Work out the finished part from the listing and answer in its coordinate system (mm). A direction names the side the tool comes from. Coordinates: 2 decimals unless noted, no trailing zeros. Write each loop counter-clockwise with the first axis right and the second up, starting at its lowest first coordinate (ties: lowest second). Pieces come first, ordered by that corner, then holes. Notation, with made-up numbers: (70.5, 60.5) - (118.5, 60.5) arc R6 cw to (118.5, 70.5) - close; hole circle Ø11 at (26.5, 38.25). An arc over 180 degrees is marked (long way). Use a Markdown table: item, result. Add a question column.
(1) A tool of negligible diameter and unlimited length cuts with its end or side. For faces 4 (the face through (1, 1, 1)), 5 (the face through (-2, 3.9, 2)), 6 (the face through (0.736, 2.683, 2.337)), from which of +Z, -Z, +X, -X, +Y, -Y can it reach the whole face along a straight path? Write none if from no direction.
(2) For a pull along Z with two mould halves and no side action, classify faces 1 (the face through (7, 0, 0)), 2 (the face through (17.2, 0.7, 0)), 3 (the face through (-1, 1.5, -1)) as released by +Z, released by -Z, zero draft, split by the parting line, or undercut.
(3) The part is cut by section B-B, the plane y = 0.4. State how many separate pieces and enclosed holes the cut face has, then the cut area to 3 significant figures.
(4) Given pin 1 Ø4 at (x, z) = (0, 0) entering from -Y; pin 2 Ø1.8 at (x, z) = (10, 0) entering from +Y; pin 3 Ø1.5 at (x, y) = (7, 1.5) entering from +Z, each flat-ended and moving along its own axis, determine where each tip first touches the part or whether it passes through.
(5) The part is cut by section D-D, the plane z = -1.5. Give the vertices of the cut face in (x, y), then the cut area to 3 significant figures.
(6) Find the intervals of material crossed by line 1 (X direction, y = 2.25, z = 1); line 2 (Y direction, x = 8.75, z = 0); line 3 (X direction, y = 0.65, z = 1.25), in increasing order. Write a range as from..to.
(7) The part is cut by section C-C, the plane z = 1. Give the vertices of the cut face in (x, y), then the cut area to 3 significant figures.
(8) The part is cut by section A-A, the plane x = 9.8. Give the vertices of the cut face in (y, z), then the cut area to 3 significant figures.
from build123d import *

# Parameters (mm, degrees)
SKETCH1_R           = 0.5
BOSS_EXTRUDE1_DEPTH = 1.4
SKETCH2_R           = 2.35
CUT_EXTRUDE1_DEPTH  = 1
SKETCH3_R           = 3.5
SKETCH3_R_2         = 2.45
BOSS_EXTRUDE2_DEPTH = 2.5
SKETCH4_R           = 1.2
CUT_EXTRUDE2_DEPTH  = 20.282440198
SKETCH5_R           = 2.45
SKETCH5_R_2         = 1.2
BOSS_EXTRUDE3_DEPTH = 0.1
SKETCH6_W           = 35.735260114
SKETCH6_H           = 17.672039004
CUT_EXTRUDE4_DEPTH  = 20.513392837
CUT_EXTRUDE5_DEPTH  = 18.980545042
SKETCH8_W           = 0.114102852
SKETCH8_H           = 0.1
CUT_EXTRUDE6_DEPTH  = 0.1


with BuildPart() as part:
    # Sketch1 → Boss-Extrude1 (new body)
    with BuildSketch(Plane(origin=(0, 0, 0), x_dir=(1, 0, 0), z_dir=(0, 1, 0))):
        with BuildLine():
            Line((-15.2, 2), (-2, 2.95))
            Line((-2, 2.95), (-2, 6.35))
            ThreePointArc((-2, 6.35), (0, 8.35), (2, 6.35))
            Line((2, 6.35), (2, 3.5))
            Line((2, 3.5), (15.2, 2))
            ThreePointArc((15.2, 2), (17.2, 0), (15.2, -2))
            Line((15.2, -2), (2, -3.5))
            Line((2, -3.5), (2, -6.35))
            ThreePointArc((2, -6.35), (0, -8.35), (-2, -6.35))
            Line((-2, -6.35), (-2, -2.95))
            Line((-2, -2.95), (-15.2, -2))
            ThreePointArc((-15.2, -2), (-17.2, 0), (-15.2, 2))
        make_face()
        with Locations(Location((0, 6.35, 0), (0, 0, 270))):
            Circle(SKETCH1_R, mode=Mode.SUBTRACT)
        with Locations(Location((0, 4.55, 0), (0, 0, 270))):
            Circle(SKETCH1_R, mode=Mode.SUBTRACT)
        with Locations(Location((0, -4.55, 0), (0, 0, 90))):
            Circle(SKETCH1_R, mode=Mode.SUBTRACT)
        with Locations(Location((0, -6.35, 0), (0, 0, 90))):
            Circle(SKETCH1_R, mode=Mode.SUBTRACT)
        with Locations(Location((-15.2, 0, 0), (0, 0, 270))):
            Circle(SKETCH1_R, mode=Mode.SUBTRACT)
        with Locations(Location((15.2, 0, 0), (0, 0, 270))):
            Circle(SKETCH1_R, mode=Mode.SUBTRACT)
        with Locations(Location((-13.4, 0, 0), (0, 0, 270))):
            Circle(SKETCH1_R, mode=Mode.SUBTRACT)
        with Locations(Location((-11.6, 0, 0), (0, 0, 270))):
            Circle(SKETCH1_R, mode=Mode.SUBTRACT)
        with Locations(Location((-9.8, 0, 0), (0, 0, 270))):
            Circle(SKETCH1_R, mode=Mode.SUBTRACT)
        with Locations(Location((-8, 0, 0), (0, 0, 270))):
            Circle(SKETCH1_R, mode=Mode.SUBTRACT)
        with Locations(Location((-6.2, 0, 0), (0, 0, 270))):
            Circle(SKETCH1_R, mode=Mode.SUBTRACT)
        with Locations(Location((-4.4, 0, 0), (0, 0, 270))):
            Circle(SKETCH1_R, mode=Mode.SUBTRACT)
        with Locations(Location((13.4, 0, 0), (0, 0, 270))):
            Circle(SKETCH1_R, mode=Mode.SUBTRACT)
        with Locations(Location((11.6, 0, 0), (0, 0, 270))):
            Circle(SKETCH1_R, mode=Mode.SUBTRACT)
        with Locations(Location((9.8, 0, 0), (0, 0, 270))):
            Circle(SKETCH1_R, mode=Mode.SUBTRACT)
        with Locations(Location((8, 0, 0), (0, 0, 270))):
            Circle(SKETCH1_R, mode=Mode.SUBTRACT)
        with Locations(Location((6.2, 0, 0), (0, 0, 270))):
            Circle(SKETCH1_R, mode=Mode.SUBTRACT)
        with Locations(Location((4.4, 0, 0), (0, 0, 270))):
            Circle(SKETCH1_R, mode=Mode.SUBTRACT)
    extrude(amount=BOSS_EXTRUDE1_DEPTH)

    # Sketch2 → Cut-Extrude1 (cut)
    with BuildSketch(Plane.XZ):
        with Locations(Location((0, 0, 0), (0, 0, 270))):
            Circle(SKETCH2_R)
    extrude(amount=-CUT_EXTRUDE1_DEPTH, mode=Mode.SUBTRACT)

    # Sketch3 → Boss-Extrude2 (add)
    with BuildSketch(Plane(origin=(0, 1.4, 0), x_dir=(1, 0, 0), z_dir=(0, 1, 0))):
        with Locations(Location((0, 0, 0), (0, 0, 270))):
            Circle(SKETCH3_R)
        with Locations(Location((0, 0, 0), (0, 0, 270))):
            Circle(SKETCH3_R_2, mode=Mode.SUBTRACT)
    extrude(amount=BOSS_EXTRUDE2_DEPTH)

    # Sketch4 → Cut-Extrude2 (cut, through all)
    with BuildSketch(Plane(origin=(0, 1.4, 0), x_dir=(1, 0, 0), z_dir=(0, 1, 0))):
        with Locations(Location((0, 0, 0), (0, 0, 270))):
            Circle(SKETCH4_R)
    extrude(amount=-CUT_EXTRUDE2_DEPTH, mode=Mode.SUBTRACT)

    # Sketch5 → Boss-Extrude3 (add)
    with BuildSketch(Plane(origin=(0, 1.4, 0), x_dir=(1, 0, 0), z_dir=(0, 1, 0))):
        with Locations(Location((0, 0, 0), (0, 0, 270))):
            Circle(SKETCH5_R)
        with Locations(Location((0, 0, 0), (0, 0, 270))):
            Circle(SKETCH5_R_2, mode=Mode.SUBTRACT)
    extrude(amount=BOSS_EXTRUDE3_DEPTH)

    # Sketch6 → Cut-Extrude4 (cut, through all)
    with BuildSketch(Plane.XZ):
        Rectangle(SKETCH6_W, SKETCH6_H)
        with BuildLine():
            Line((-1.868584713, -2.959457918), (-15.2, -2))
            ThreePointArc((-15.2, -2), (-17.2, 0), (-15.2, 2))
            Line((-15.2, 2), (-1.868584713, 2.959457918))
            ThreePointArc((-1.868584713, 2.959457918), (0, 3.5), (1.868584713, 2.959457918))
            Line((1.868584713, 2.959457918), (15.2, 2))
            ThreePointArc((15.2, 2), (17.2, 0), (15.2, -2))
            Line((15.2, -2), (1.868584713, -2.959457918))
            ThreePointArc((1.868584713, -2.959457918), (0, -3.5), (-1.868584713, -2.959457918))
        make_face(mode=Mode.SUBTRACT)
    extrude(amount=-CUT_EXTRUDE4_DEPTH, mode=Mode.SUBTRACT)

    # Sketch7 → Cut-Extrude5 (cut, through all)
    with BuildSketch(Plane.XZ):
        with BuildLine():
            Line((0, 3.5), (-17.731768104, 3.5))
            Line((-17.731768104, 3.5), (-17.731768104, -3.5))
            Line((-17.731768104, -3.5), (0, -3.5))
            ThreePointArc((0, -3.5), (-3.5, 0), (0, 3.5))
        make_face()
    extrude(amount=-CUT_EXTRUDE5_DEPTH, mode=Mode.SUBTRACT)

    # Sketch8 → Cut-Extrude6 (cut)
    with BuildSketch(Plane(origin=(0, 1.4, 0), x_dir=(1, 0, 0), z_dir=(0, 1, 0))):
        with Locations((15.857051426, 0)):
            Rectangle(SKETCH8_W, SKETCH8_H)
    extrude(amount=-CUT_EXTRUDE6_DEPTH, mode=Mode.SUBTRACT)


solid = part.part
Model answer:
| question | item | result |
|---|---|---|
| 1 | face 4 | -Y |
| 1 | face 5 | +Z, -Z, +X, -X, +Y |
| 1 | face 6 | +Y |
| 2 | face 1 | zero draft |
| 2 | face 2 | split by the parting line |
| 2 | face 3 | undercut |
| 3 | separate pieces | 1 |
| 3 | enclosed holes | 8 |
| 3 | area | 81.2 mm^2 |
| 4 | pin 1 | y = 1 |
| 4 | pin 2 | y = 1.4 |
| 4 | pin 3 | z = 2.64 |
| 5 | outline | (-3.16, 0) - (-1.81, 0) - (-1.81, 1) - (1.81, 1) - (1.81, 0) - (16.52, 0) - (16.52, 1.4) - (3.16, 1.4) - (3.16, 3.9) - (1.94, 3.9) - (1.94, 1.5) - (-1.94, 1.5) - (-1.94, 3.9) - (-3.16, 3.9) - close |
| 5 | area | 30.5 mm^2 |
| 6 | line 1 | -3.35..-2.24, 2.24..3.35 |
| 6 | line 2 | 0..1.4 |
| 6 | line 3 | -3.27..-1.99, 1.99..16.76 |
| 7 | outline | (-3.35, 0) - (-2.13, 0) - (-2.13, 1) - (-0.66, 1) - (-0.66, 1.5) - (-2.24, 1.5) - (-2.24, 3.9) - (-3.35, 3.9) - close; (0.66, 1) - (2.13, 1) - (2.13, 0) - (16.93, 0) - (16.93, 1.4) - (3.35, 1.4) - (3.35, 3.9) - (2.24, 3.9) - (2.24, 1.5) - (0.66, 1.5) - close |
| 7 | area | 29.5 mm^2 |
| 8 | outline | (0, -2.39) - (1.4, -2.39) - (1.4, -0.5) - (0, -0.5) - close; (0, 0.5) - (1.4, 0.5) - (1.4, 2.39) - (0, 2.39) - close |
| 8 | area | 5.29 mm^2 |
